```python
from build123d import *

# Parameters (mm, degrees)
F1_DEPTH  = 44
F3_R      = 4
F4_DEPTH  = 25
F6_DEPTH  = 25
F7_R      = 3
F8_R      = 10
F9_R      = 7.25
F10_DEPTH = 25


with BuildPart() as f1:
    # F0 (on Front) → F1 (new body)
    with BuildSketch(Plane.XZ):
        Polygon((0, 70), (0, 0), (3, 0), (3, 67), (33, 67), (33, 0), (36, 0), (36, 70), align=None)
    extrude(amount=F1_DEPTH)

    # F2 (on face) + F3 (on face) → F4 (cut)
    with BuildSketch(Plane.YZ.offset(36)):
        Polygon((0, 0), (0, 70), (-22, 0), align=None)
    with BuildSketch(Plane.YZ.offset(36)):
        with Locations((-34, 10)):
            Circle(F3_R)
    extrude(amount=-F4_DEPTH, mode=Mode.SUBTRACT)

    # F5 (on face) → F6 (cut)
    with BuildSketch(Plane(origin=(0, 0, 0), x_dir=(0, -1, 0), z_dir=(-1, 0, 0))):
        Polygon((22, 0), (0, 70), (0, 0), align=None)
        with BuildLine():
            Line((32.75, 16), (32.75, 13.7996710384))
            ThreePointArc((32.75, 13.7996710384), (34, 6), (35.25, 13.7996710384))
            Line((35.25, 13.7996710384), (35.25, 16))
            Line((35.25, 16), (34, 16))
            Line((34, 16), (32.75, 16))
        make_face()
    extrude(amount=-F6_DEPTH, mode=Mode.SUBTRACT)

    # F7
    f7_edges = [f1.edges().sort_by_distance(p)[0] for p in [
        (33, -22.471429, 67),
        (3, -22.471429, 67),
        (36, -22, 70),
        (0, -22, 70),
    ]]
    fillet(f7_edges, radius=F7_R)

    # F8
    f8_edges = [f1.edges().sort_by_distance(p)[0] for p in [
        (1.5, -44, 0),
        (34.5, -44, 0),
        (1.5, -22, 0),
        (34.5, -22, 0),
    ]]
    fillet(f8_edges, radius=F8_R)

    # F9 (on face) → F10 (cut)
    with BuildSketch(Plane.XY.offset(70)):
        with Locations((18, -22)):
            Circle(F9_R)
    extrude(amount=-F10_DEPTH, mode=Mode.SUBTRACT)


solid = f1.part
```
Check sheet for the modelled part. Datum: model origin and axes. Units: mm. A direction names the side the tool comes from. Give positions to 0.01 mm unless a question says otherwise; leave off trailing zeros. Write each loop counter-clockwise with the first axis right and the second up, starting at its lowest first coordinate (ties: lowest second). Pieces come first, ordered by that corner, then holes. Notation, with made-up numbers: (77, -38) -> (116, -38) arc R12 ccw to (116, -29) -> close; hole circle Ø5 at (81.5, 21). An arc over 180 degrees is marked (long way). Use CSV: the item, a comma, the result in double quotes. Start each with the question number.
Q1. Release check for a two-part mould opening along Z. For faces 1 (the cylindrical face through (0.86, -22.31, 69.1)), 2 (the flat face through (1, -34, 16)), 3 (the flat face through (1, -32, 0)) record: +Z half, -Z half, draft (parallel to the pull), parting line (faces both ways), or undercut.
Q2. Scan lines: line 1 along X through (y, z) = (-30, 28); line 2 along Z through (x, y) = (29, -20.5); line 3 along Z through (x, y) = (1.4, -34). Record each from-to range of solid material in increasing order.
Q3. Cross-section at B-B on x = 18. Enter the section's corners in (y, z).
Q4. Tool access check on faces 4 (the flat face through (1, -32.75, 15)), 5 (the cylindrical face through (34.52, -41.15, 3.01)), 6 (the cylindrical face through (32.1, -22.77, 66.14)). Record the directions out of +Z, -Z, +X, -X, +Y, -Y that give a thin tool (end or side, any length) a straight path to the whole face; none if there is none.
Q5. Cross-section at A-A on z = 52.5. Enter the section's corners in (x, y), and give its area (3 significant figures).
Q6. Cross-section at D-D on z = 8. Enter the section's corners in (x, y).
Q7. Cross-section at C-C on y = -22. Enter the section's corners in (x, z), and give its area (3 significant figures).
Q8. Depth check by flat-ended pin: P1, Ø0.7, axis at x = 1.5, z = 14.5, coming from the +Y side; P2, Ø16.5, axis at x = 18, y = -22, coming from the -Z side; P3, Ø12, axis at x = 6, z = 26.5, coming from the +Y side. Enter the tip coordinate at first touch or a pass-through.
Working result:
1,face 1,"+Z half"
1,face 2,"undercut"
1,face 3,"-Z half"
2,line 1,"x = 0 to 3, 33 to 36"
2,line 2,"z = 67 to 70"
2,line 3,"z = 0 to 6, 16 to 69.54"
3,outline,"(-44, 67) -> (-29.25, 67) -> (-29.25, 70) -> (-44, 70) -> close; (-14.75, 67) -> (-0.94, 67) -> (0, 70) -> (-14.75, 70) -> close"
4,face 4,"-X"
4,face 5,"-Z, +X, -X, -Y"
4,face 6,"-Z, +Y, -Y"
5,outline,"(0, -44) -> (3, -44) -> (3, -5.5) -> (0, -5.5) -> close; (33, -44) -> (36, -44) -> (36, -5.5) -> (33, -5.5) -> close"
5,area,"231 mm^2"
6,outline,"(0, -43.8) -> (3, -43.8) -> (3, -37.46) -> (0, -37.46) -> close; (0, -30.54) -> (3, -30.54) -> (3, -19.49) -> (0, -19.49) -> close; (33, -43.8) -> (36, -43.8) -> (36, -37.46) -> (33, -37.46) -> close; (33, -30.54) -> (36, -30.54) -> (36, -19.49) -> (33, -19.49) -> close"
7,outline,"(0, 3.21) -> (3, 3.21) -> (3, 64) arc R3 cw to (6, 67) -> (10.75, 67) -> (10.75, 70) -> (3, 70) arc R3 ccw to (0, 67) -> close; (25.25, 67) -> (30, 67) arc R3 cw to (33, 64) -> (33, 3.21) -> (36, 3.21) -> (36, 67) arc R3 ccw to (33, 70) -> (25.25, 70) -> close"
7,area,"447 mm^2"
8,P1,"stops at y = -17.33"
8,P2,"stops at z = 67"
8,P3,"stops at y = -12.04"
